```python
from build123d import *

# Parameters (mm, degrees)
BOSS_EXTRUDE1_DEPTH   = 0.9
BOSS_EXTRUDE2_DEPTH   = 17.1
FILLET2_R             = 1
FILLET3_R             = 0.2
SKETCH4_R             = 5
CUT_EXTRUDE1_DEPTH    = 8
M8_TAPPED_HOLE1_D     = 6.8
M8_TAPPED_HOLE1_DEPTH = 22.25
M8_TAPPED_HOLE1_TIP   = 2.042926105
CHAMFER1_SIZE         = 0.5


with BuildPart() as part:
    # Sketch1 → Boss-Extrude1 (new body)
    with BuildSketch(Plane(origin=(0, 0, 0), x_dir=(1, 0, 0), z_dir=(0, 1, 0))):
        Polygon((6.92820323, 0), (3.464101615, 6), (-3.464101615, 6), (-6.92820323, 0), (-3.464101615, -6), (3.464101615, -6), align=None)
    extrude(amount=-BOSS_EXTRUDE1_DEPTH)

    # Sketch2 → Boss-Extrude2 (add)
    with BuildSketch(Plane.XZ.offset(0.9)):
        Polygon((-6.293117934, 0), (-3.146558967, -5.45), (3.146558967, -5.45), (6.293117934, 0), (3.146558967, 5.45), (-3.146558967, 5.45), align=None)
    extrude(amount=BOSS_EXTRUDE2_DEPTH)

    # Sketch3 → Cut-Revolve1 (revolve, cut)
    with BuildSketch(Plane.XY, mode=Mode.PRIVATE) as cut_revolve1_sk:
        Polygon((-6.293117934, -18), (-5.25, -18), (-6.293117934, -14), align=None)
    revolve(cut_revolve1_sk.sketch.rotate(Axis((0, 0, 0), (0, -1, 0)), 270), axis=Axis((0, 0, 0), (0, -1, 0)), mode=Mode.SUBTRACT)

    # Fillet2
    fillet2_edges = [part.edges().sort_by_distance(p)[0] for p in [
        (-6.92820323, -0.45, 0),
        (-6.293117934, -7.45, 0),
        (-3.146558967, -7.45, -5.45),
        (-3.464101615, -0.45, -6),
        (3.146558967, -7.45, -5.45),
        (3.464101615, -0.45, -6),
        (6.293117934, -7.45, 0),
        (6.92820323, -0.45, 0),
        (3.146558967, -7.45, 5.45),
        (3.464101615, -0.45, 6),
        (-3.146558967, -7.45, 5.45),
        (-3.464101615, -0.45, 6),
    ]]
    fillet(fillet2_edges, radius=FILLET2_R)

    # Fillet3
    fillet3_edges = [part.edges().sort_by_distance(p)[0] for p in [
        (-3.069208698, -0.9, -5.316025404),
        (3.069208698, -0.9, -5.316025404),
        (6.138417396, -0.9, 0),
        (3.069208698, -0.9, 5.316025404),
        (-3.069208698, -0.9, 5.316025404),
        (-6.138417396, -0.9, 0),
        (0, -0.9, -5.45),
        (-4.719838451, -0.9, -2.725),
        (-4.719838451, -0.9, 2.725),
        (0, -0.9, 5.45),
        (4.719838451, -0.9, 2.725),
        (4.719838451, -0.9, -2.725),
    ]]
    fillet(fillet3_edges, radius=FILLET3_R)

    # Sketch4 → Cut-Extrude1 (cut)
    with BuildSketch(Plane(origin=(0, 0, 0), x_dir=(1, 0, 0), z_dir=(0, 1, 0))):
        with Locations(Location((0, 0, 0), (0, 0, 270))):
            Circle(SKETCH4_R)
    extrude(amount=-CUT_EXTRUDE1_DEPTH, mode=Mode.SUBTRACT)

    # M8 Tapped Hole1
    with Locations(Plane(origin=(0, -8, 0), x_dir=(1, 0, 0), z_dir=(0, 1, 0))):
        with Locations((0, 0)):
            Hole(M8_TAPPED_HOLE1_D / 2, depth=M8_TAPPED_HOLE1_DEPTH)
            with Locations((0, 0, -(M8_TAPPED_HOLE1_DEPTH + M8_TAPPED_HOLE1_TIP / 2))):  # 118° drill point
                Cone(0, M8_TAPPED_HOLE1_D / 2, M8_TAPPED_HOLE1_TIP, mode=Mode.SUBTRACT)

    # Chamfer1
    chamfer1_edges = [part.edges().sort_by_distance(p)[0] for p in [
        (3.4, -18, 0),
        (3.4, -8, 0),
    ]]
    chamfer(chamfer1_edges, length=CHAMFER1_SIZE)


solid = part.part
```
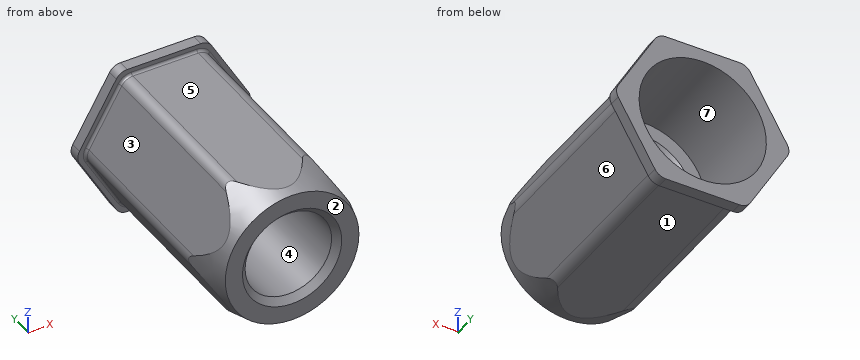
For this review, take the finished solid that the model builds, in its own axes (mm). Face numbers are marked on the shaded views. A direction names the side the tool comes from. Coordinates: 2 decimals unless noted, no trailing zeros. Write each loop counter-clockwise with the first axis right and the second up, starting at its lowest first coordinate (ties: lowest second). Pieces come first, ordered by that corner, then holes. Notation, with made-up numbers: (71.25, 23) - (85.25, 23) arc R20 ccw to (85.25, 49) - close; hole circle Ø5 at (-22, 55.5). An arc over 180 degrees is marked (long way). Answer in a Markdown table with one row per item. Add a question column.
Q1. We need section A-A, the plane y = -2. State the section outline as (x, z) points, and give its area (3 significant figures).
Q2. We need section D-D, the plane y = -11.5. State the section outline as (x, z) points.
Q3. We need section C-C, the plane x = 0. State the section outline as (y, z) points.
Q4. We need section B-B, the plane z = 0. State the section outline as (x, y) points.
Q5. For probe 1 along Z at (x, y) = (0, -15); probe 2 along X at (y, z) = (-13.5, 0); probe 3 along X at (y, z) = (-2, -1.5), list the stretches that pass through material, from the lowest coordinate up.
Q6. Tool access review of the marked faces 1, 2 and 3: name each direction out of +Z, -Z, +X, -X, +Y, -Y from which nothing blocks a thin tool from reaching the whole face with its end or side.
Q7. For P1, Ø3, axis at y = -12.5, z = -4, coming from the -X side; P2, Ø2.5, axis at x = 1, y = -7, coming from the +Z side; P3, Ø5.5, axis at x = 0, z = 0, coming from the -Y side; P4, Ø3, axis at x = -2.5, z = -1.5, coming from the +Y side, all flat-tipped, find the tip position at first contact; note any pin that passes through.
Q8. Draft analysis for pull direction X (two halves, no side actions). For the marked faces 4, 5, 6 and 7, state which applies: +X half, -X half, draft (parallel to the pull), parting line (faces both ways), or undercut.
Answer list:
| question | item | result |
|---|---|---|
| 1 | outline | (-6, -0.5) - (-3.44, -4.95) arc R1 ccw to (-2.57, -5.45) - (2.57, -5.45) arc R1 ccw to (3.44, -4.95) - (6, -0.5) arc R1 ccw to (6, 0.5) - (3.44, 4.95) arc R1 ccw to (2.57, 5.45) - (-2.57, 5.45) arc R1 ccw to (-3.44, 4.95) - (-6, 0.5) arc R1 ccw to start; hole circle Ø10 at (0, 0) |
| 1 | area | 24.0 mm2 |
| 2 | outline | (-6, -0.5) - (-3.44, -4.95) arc R1 ccw to (-2.57, -5.45) - (2.57, -5.45) arc R1 ccw to (3.44, -4.95) - (6, -0.5) arc R1 ccw to (6, 0.5) - (3.44, 4.95) arc R1 ccw to (2.57, 5.45) - (-2.57, 5.45) arc R1 ccw to (-3.44, 4.95) - (-6, 0.5) arc R1 ccw to start; hole circle Ø6.8 at (0, 0) |
| 3 | outline | (-18, -5.25) - (-17.23, -5.45) - (-1.1, -5.45) arc R0.2 cw to (-0.9, -5.65) - (-0.9, -6) - (0, -6) - (0, -5) - (-8, -5) - (-8, -3.9) - (-8.5, -3.4) - (-17.5, -3.4) - (-18, -3.9) - close; (-18, 3.9) - (-17.5, 3.4) - (-8.5, 3.4) - (-8, 3.9) - (-8, 5) - (0, 5) - (0, 6) - (-0.9, 6) - (-0.9, 5.65) arc R0.2 cw to (-1.1, 5.45) - (-17.23, 5.45) - (-18, 5.25) - close |
| 4 | outline | (-6.77, -0.9) - (-6.34, -0.9) arc R0.2 cw to (-6.14, -1.1) - (-6.14, -14.59) - (-5.25, -18) - (-3.9, -18) - (-3.4, -17.5) - (-3.4, -8.5) - (-3.9, -8) - (-5, -8) - (-5, 0) - (-6.77, 0) - close; (3.4, -17.5) - (3.9, -18) - (5.25, -18) - (6.14, -14.59) - (6.14, -1.1) arc R0.2 cw to (6.34, -0.9) - (6.77, -0.9) - (6.77, 0) - (5, 0) - (5, -8) - (3.9, -8) - (3.4, -8.5) - close |
| 5 | probe 1 | z = -5.45 to -3.4, 3.4 to 5.45 |
| 5 | probe 2 | x = -6.14 to -3.4, 3.4 to 6.14 |
| 5 | probe 3 | x = -5.43 to -4.77, 4.77 to 5.43 |
| 6 | face 1 | -Z, +X, -X, -Y |
| 6 | face 2 | +Z, -Z, +X, -X, -Y |
| 6 | face 3 | +Z, -X, -Y |
| 7 | P1 | stops at x = -4.85 |
| 7 | P2 | stops at z = 5.45 |
| 7 | P3 | passes through |
| 7 | P4 | stops at y = -8 |
| 8 | face 4 | undercut |
| 8 | face 5 | draft |
| 8 | face 6 | +X half |
| 8 | face 7 | undercut |
